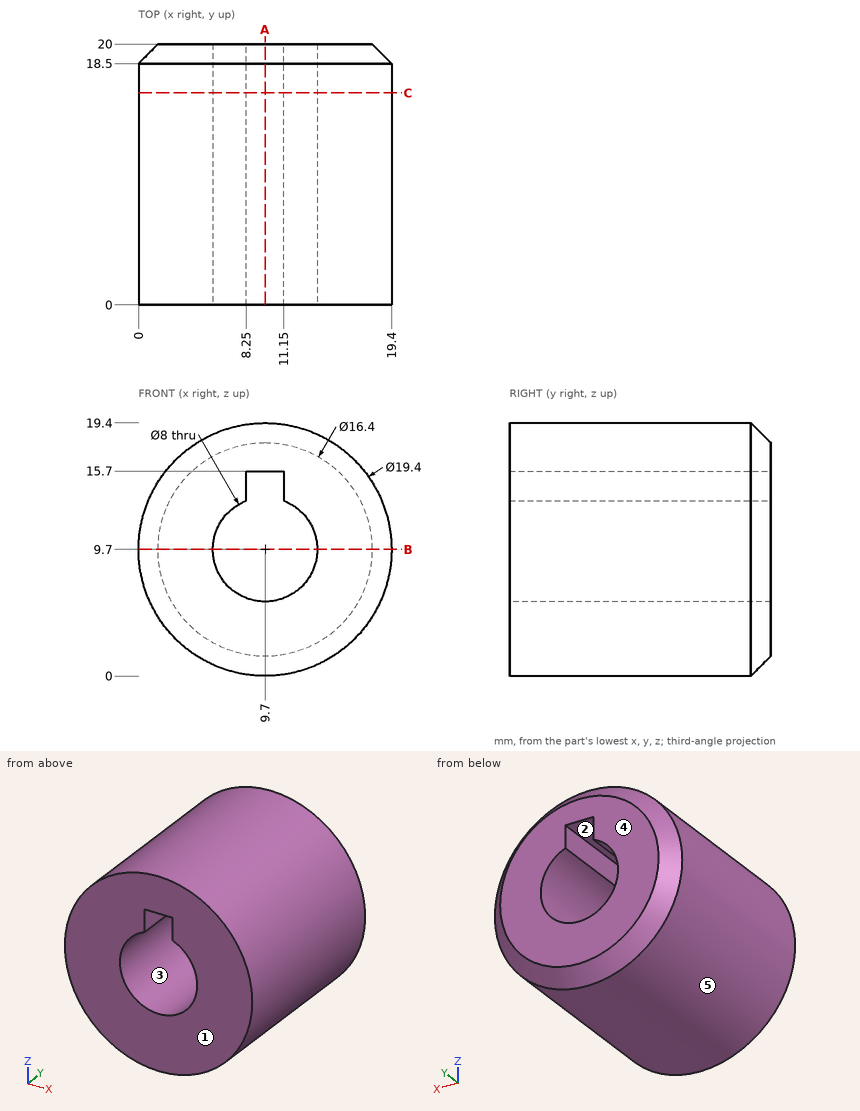
Part print with two shaded views. Sizes in mm from the minimum x, y, z corner. A direction names the side the tool comes from. Coordinates: 2 decimals unless noted, no trailing zeros. Write each loop counter-clockwise with the first axis right and the second up, starting at its lowest first coordinate (ties: lowest second). Pieces come first, ordered by that corner, then holes.
1. Band-saw the part on B-B, the plane z = 9.7. Give the cut face in (x, y), and give its area (3 significant figures).
Answer block:
outline: (0, 0) - (5.7, 0) - (5.7, 20) - (1.5, 20) - (0, 18.5) - close; (13.7, 0) - (19.4, 0) - (19.4, 18.5) - (17.9, 20) - (13.7, 20) - close
area: 226 mm2
2. 3-axis set-ups, long thin cutter, end or side, ignore diameter. For the marked faces 1 and 2: which of +Z, -Z, +X, -X, +Y, -Y reach the whole face in a straight line?
Answer block:
face 1: +Z, -Z, +X, -X, -Y
face 2: +Y, -Y
3. Pull direction Z, two halves, no side cores. Call the marked faces 3, 4 and 5: released by +Z, released by -Z, zero draft, split by the parting line, or undercut.
Answer block:
face 3: undercut
face 4: zero draft
face 5: split by the parting line
4. Drill centre lines: probe 1 along X at (y, z) = (11.75, 9.7); probe 2 along Z at (x, y) = (9.5, 16.25) (3 decimals); probe 3 along X at (y, z) = (6.75, 10.75). Where is each one in solid material? Low to high.
Answer block:
probe 1: x = 0 to 5.7, 13.7 to 19.4
probe 2: z = 0.002 to 5.705, 15.7 to 19.398
probe 3: x = 0.06 to 5.84, 13.56 to 19.34
5. Band-saw the part on A-A, the plane x = 9.7. Give the cut face in (y, z), and give its area (3 significant figures).
Answer block:
outline: (0, 0) - (18.5, 0) - (20, 1.5) - (20, 5.7) - (0, 5.7) - close; (0, 15.7) - (20, 15.7) - (20, 17.9) - (18.5, 19.4) - (0, 19.4) - close
area: 186 mm2
6. Drop flat-ended pins along their axis: pin 1 (2 mm diameter, centred on x = 4.5, y = 8.5, fed in from +Z); pin 2 (3 mm diameter, centred on y = 17, z = 6.5, fed in from +X); pin 3 (2.5 mm diameter, centred on y = 14, z = 15, fed in from -X). Give the stop position or say it passes through.
Answer block:
pin 1: stops at z = 18.44
pin 2: stops at x = 19.25
pin 3: stops at x = 0.89
7. Band-saw the part on C-C, the plane y = 16.25. Give the cut face in (x, z).
Answer block:
outline: circle Ø19.4 at (9.7, 9.7); hole (8.25, 13.43) arc R4 ccw (long way) to (11.15, 13.43) - (11.15, 15.7) - (8.25, 15.7) - close
